from build123d import *

# Parameters (mm, degrees)
SKETCH1_R           = 2.75
BOSS_EXTRUDE1_DEPTH = 4
FILLET1_R           = 1


with BuildPart() as part:
    # Sketch1 → Boss-Extrude1 (new body)
    with BuildSketch(Plane.XY):
        with BuildLine():
            Line((-12.318854252, -2.75), (12.318854252, -2.75))
            ThreePointArc((12.318854252, -2.75), (15.090593721, -3.104932583), (17.683463981, -4.146825397))
            ThreePointArc((17.683463981, -4.146825397), (24.75, 0), (17.683463981, 4.146825397))
            ThreePointArc((17.683463981, 4.146825397), (15.090593721, 3.104932583), (12.318854252, 2.75))
            Line((12.318854252, 2.75), (-12.318854252, 2.75))
            ThreePointArc((-12.318854252, 2.75), (-15.090593721, 3.104932583), (-17.683463981, 4.146825397))
            ThreePointArc((-17.683463981, 4.146825397), (-24.75, 0), (-17.683463981, -4.146825397))
            ThreePointArc((-17.683463981, -4.146825397), (-15.090593721, -3.104932583), (-12.318854252, -2.75))
        make_face()
        with Locations((-20, 0)):
            Circle(SKETCH1_R, mode=Mode.SUBTRACT)
        with Locations((20, 0)):
            Circle(SKETCH1_R, mode=Mode.SUBTRACT)
    extrude(amount=BOSS_EXTRUDE1_DEPTH)

    # Fillet1
    fillet1_edges = [part.edges().sort_by_distance(p)[0] for p in [
        (15.090593721, 3.104932583, 0),
        (24.75, 0, 0),
        (15.090593721, -3.104932583, 0),
        (0, -2.75, 0),
        (24.75, 0, 4),
        (15.090593721, 3.104932583, 4),
        (0, 2.75, 4),
        (-15.090593721, 3.104932583, 4),
        (-24.75, 0, 4),
        (-15.090593721, -3.104932583, 4),
        (0, -2.75, 4),
        (-15.090593721, -3.104932583, 0),
        (15.090593721, -3.104932583, 4),
        (-24.75, 0, 0),
        (-15.090593721, 3.104932583, 0),
        (0, 2.75, 0),
    ]]
    fillet(fillet1_edges, radius=FILLET1_R)


solid = part.part
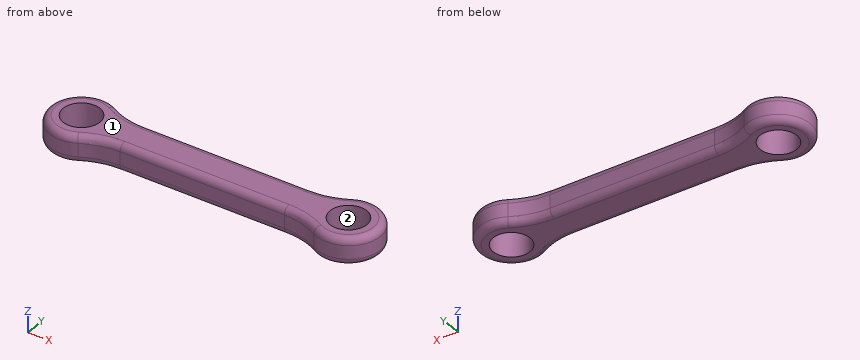
Input: part model. Units: mm. Frame: model coordinates. Face numbers are marked on the shaded views. Coordinates: 2 decimals unless noted, no trailing zeros. Write each loop counter-clockwise with the first axis right and the second up, starting at its lowest first coordinate (ties: lowest second). Pieces come first, ordered by that corner, then holes. Notation, with made-up numbers: M -21.5,-18 L 37.5,-18 A11 ccw 37.5,1 Z; hole C 29.25,-27 d7. An arc over 180 degrees is marked long. Answer as a JSON object with one key per item and string values. Group by question number.
(1) Mould query, pull axis X, two halves, no side actions, for the marked faces 1 and 2. Classes: pulls with the +X half, pulls with the -X half, needs draft (parallel to the pull), parting line crosses it, or undercut.
(2) Section A-A on y = 0. Output: boundary loops of the cut face in (x, z), plus the area to 3 significant figures.
(3) Contact query for flat-ended pins moving along their axis: P1, Ø1.6, axis at x = -3, z = 2, coming from the -Y side; P2, Ø1, axis at x = -2.5, z = 2, coming from the +Y side; P3, Ø2, axis at y = -3, z = 2.5, coming from the -X side. Output: stop coordinate, or through.
(4) Ray query, line 1 along X through (y, z) = (-1.5, 1.05); line 2 along X through (y, z) = (-1.5, 3.5); line 3 along Y through (x, z) = (-20, 2.65). Return the intervals inside material, ascending. Write a range as [from, to].
(5) Section B-B on x = -9.5. Output: boundary loops of the cut face in (y, z).
Result set:
{
 "1": {"face 1": "needs draft", "face 2": "undercut"},
 "2": {"outline": "M -24.75,1 A1 ccw -23.75,0 L -22.75,0 L -22.75,4 L -23.75,4 A1 ccw -24.75,3 Z; M -17.25,0 L 17.25,0 L 17.25,4 L -17.25,4 Z; M 22.75,0 L 23.75,0 A1 ccw 24.75,1 L 24.75,3 A1 ccw 23.75,4 L 22.75,4 Z", "area": "153 mm2"},
 "3": {"P1": "stops at y = -2.75", "P2": "stops at y = 2.75", "P3": "stops at x = -24.31"},
 "4": {"line 1": "x = [-24.51, -22.3], [-17.7, 17.7], [22.3, 24.51]", "line 2": "x = [-24.37, -22.3], [-17.7, 17.7], [22.3, 24.37]", "line 3": "y = [-4.75, -2.75], [2.75, 4.75]"},
 "5": {"outline": "M -2.75,1 A1 ccw -1.75,0 L 1.75,0 A1 ccw 2.75,1 L 2.75,3 A1 ccw 1.75,4 L -1.75,4 A1 ccw -2.75,3 Z"}
}
